```python
from build123d import *

# Parameters (mm, degrees)
F0_R      = 14
F1_DEPTH  = 159
F3_W      = 18
F3_H      = 216
F4_DEPTH  = 19
F3_W_2    = 14
F3_H_2    = 4.5
F5_DEPTH  = 18
F7_W      = 20
F7_H      = 29
F7_H_2    = 25
F7_H_3    = 23
F8_DEPTH  = 8.6
F3_W_3    = 11
F3_H_3    = 32
F9_DEPTH  = 10
F13_R     = 10.5
F14_DEPTH = 11
F11_R     = 5
F15_DEPTH = 318
F13_R_2   = 11.25
F16_DEPTH = 4
F17_DEPTH = 20


with BuildPart() as f1:
    # F0 (on Top) → F1 (new body, symmetric)
    with BuildSketch(Plane.XY):
        Circle(F0_R)
    extrude(amount=F1_DEPTH, both=True)

    # F3 (on offset) → F4 (cut)
    with BuildSketch(Plane.YZ.offset(14)):
        with Locations((0, -28)):
            Rectangle(F3_W, F3_H)
    extrude(amount=-F4_DEPTH, mode=Mode.SUBTRACT)

    # F3 (on offset) → F5 (cut)
    with BuildSketch(Plane.YZ.offset(14)):
        with Locations((0, -141.25)):
            Rectangle(F3_W_2, F3_H_2)
    extrude(amount=-F5_DEPTH, mode=Mode.SUBTRACT)

    # F7 (on offset) → F8 (cut)
    with BuildSketch(Plane.YZ.offset(-14)):
        Polygon((-10, -98), (-10, -136), (-2.5, -136), (2.5, -136), (10, -136), (10, -98), align=None)
        with Locations((0, -60.5)):
            Rectangle(F7_W, F7_H)
        with Locations((0, -10.5)):
            Rectangle(F7_W, F7_H_2)
        Polygon((-10, 47), (-10, 25), (10, 25), (10, 47), (2.5, 47), (-2.5, 47), align=None)
        with Locations((0, -86.5)):
            Rectangle(F7_W, F7_H_3)
        with Locations((0, -34.5)):
            Rectangle(F7_W, F7_H_3)
        with Locations((0, 13.5)):
            Rectangle(F7_W, F7_H_3)
        Polygon((-10, 97), (-10, 47), (-2.5, 47), (2.5, 47), (10, 47), (10, 97), align=None)
    extrude(amount=F8_DEPTH, mode=Mode.SUBTRACT)

    # F3 (on offset) → F9 (cut)
    with BuildSketch(Plane.YZ.offset(14)):
        with Locations((0, 126)):
            Rectangle(F3_W_3, F3_H_3)
    extrude(amount=-F9_DEPTH, mode=Mode.SUBTRACT)

    # F13 (on offset) → F14 (cut)
    with BuildSketch(Plane.XY.offset(-159)):
        Circle(F13_R)
    extrude(amount=F14_DEPTH, mode=Mode.SUBTRACT)

    # F11 (on offset) → F15 (cut)
    with BuildSketch(Plane.XY.offset(159)):
        Circle(F11_R)
    extrude(amount=-F15_DEPTH, mode=Mode.SUBTRACT)

    # F13 (on offset) → F16 (cut)
    with BuildSketch(Plane.XY.offset(-159)):
        Circle(F13_R_2)
        Circle(F13_R, mode=Mode.SUBTRACT)
    extrude(amount=F16_DEPTH, mode=Mode.SUBTRACT)

    # F13 (on offset) → F17 (cut)
    with BuildSketch(Plane.XY.offset(-159)):
        with BuildLine():
            ThreePointArc((-7.2111025509, -12), (-3.7416573868, -13.4907375632), (0, -14))
            Line((0, -14), (0, -12))
            Line((0, -12), (-7.2111025509, -12))
        make_face()
        with BuildLine():
            ThreePointArc((0, -14), (3.7416573868, -13.4907375632), (7.2111025509, -12))
            Line((7.2111025509, -12), (0, -12))
            Line((0, -12), (0, -14))
        make_face()
        with BuildLine():
            Line((-7.2111025509, 12), (7.2111025509, 12))
            ThreePointArc((7.2111025509, 12), (0, 14), (-7.2111025509, 12))
        make_face()
    extrude(amount=F17_DEPTH, mode=Mode.SUBTRACT)


solid = f1.part
```
Geometry check sheet. Reference: the model listing, model coordinates, mm. A direction names the side the tool comes from. Round coordinates to 2 decimals unless told otherwise and drop trailing zeros. Order: outer loops, then holes, each group sorted by start corner. A loop starts at its lowest first (then second) coordinate and runs counter-clockwise, first axis right, second up. Notation, with made-up numbers: (84, -32) - (131, -32) arc R9 ccw to (131, -19) - close; hole circle Ø10 at (86, 87). An arc over 180 degrees is marked (long way). Use a Markdown table: item, result. Add a question column.
1) Section check B-B (z = 136.5). Record the cut outline in (x, y).
2) Thickness scan on line 1 along Z through (x, y) = (12, 1); line 2 along Z through (x, y) = (4.25, 4.5); line 3 along Z through (x, y) = (-8.75, -7.5). Record the ranges inside material, lowest first.
3) Mould release check, pull along Y, two halves, no side actions. Record for faces 1 (the cylindrical face through (-5, 0, 120)), 2 (the flat face through (0, -12, -149)), 3 (the flat face through (0, -6, 159)), 4 (the flat face through (-9, 0, 97)): released by +Y, released by -Y, zero draft, split by the parting line, or undercut.
4) Gauge pin test, flat ends, axial feed: P1, Ø2, axis at x = -1.5, z = -46.5, coming from the -Y side; P2, Ø3.5, axis at x = 1, z = -141.5, coming from the +Y side; P3, Ø5, axis at x = -7.5, z = -70, coming from the -Y side. Record the tip position at first contact, or that the pin passes through.
5) Set-up check for faces 5 (the flat face through (5, -2, -148)), 6 (the flat face through (-9, 0, -136)), 7 (the cylindrical face through (-5, 0, -142)), 8 (the flat face through (8, -5.5, 126)): record each of +Z, -Z, +X, -X, +Y, -Y from which the full face is reachable in a straight line by a thin tool's end or side.
6) Section check A-A (z = -103). Record the cut outline in (x, y).
Established:
| question | item | result |
|---|---|---|
| 1 | outline | (4, -5.5) - (4, -3) arc R5 cw (long way) to (4, 3) - (4, 5.5) - (12.87, 5.5) arc R14 ccw (long way) to (12.87, -5.5) - close |
| 2 | line 1 | -159 to -143.5, -139 to -136, 80 to 110, 142 to 159 |
| 2 | line 2 | -148 to -143.5, -139 to -136, 80 to 110, 142 to 159 |
| 2 | line 3 | -159 to -136, 97 to 159 |
| 3 | face 1 | undercut |
| 3 | face 2 | released by -Y |
| 3 | face 3 | zero draft |
| 3 | face 4 | undercut |
| 4 | P1 | y = -13.99 |
| 4 | P2 | y = 12 |
| 4 | P3 | y = -13.08 |
| 5 | face 5 | -Z |
| 5 | face 6 | -X |
| 5 | face 7 | +Z, -Z |
| 5 | face 8 | +X |
| 6 | outline | (-9.8, -10) arc R14 ccw to (10.72, -9) - (-5, -9) - (-5, 9) - (10.72, 9) arc R14 ccw to (-9.8, 10) - (-5.4, 10) - (-5.4, -10) - close |
